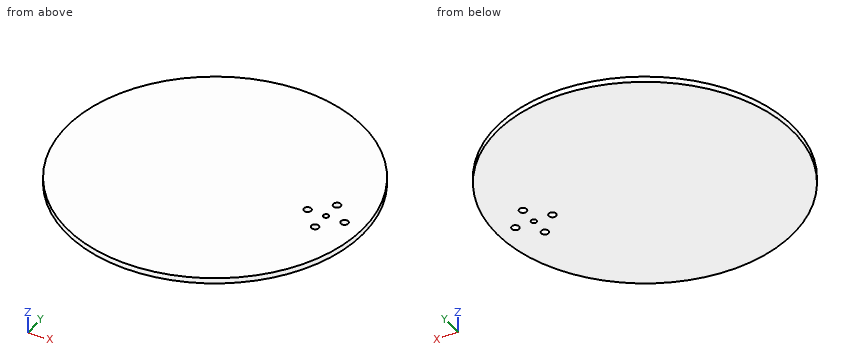
from build123d import *

# Parameters (mm, degrees)
SKETCH_1_R          = 80
EXTRUDE_1_DEPTH     = 3
SKETCH_2_R          = 2
SKETCH_2_R_2        = 1.5
CUT_EXTRUDE_4_DEPTH = 3


with BuildPart() as part:
    # 草图1 → 凸台-拉伸1 (new body)
    with BuildSketch(Plane.XY):
        Circle(SKETCH_1_R)
    extrude(amount=EXTRUDE_1_DEPTH)

    # 草图2 → 切除-拉伸4 (cut)
    with BuildSketch(Plane.XY.offset(3)):
        with Locations((70, 0)):
            Circle(SKETCH_2_R)
        with Locations((60, -10)):
            Circle(SKETCH_2_R)
        with Locations((60, 0)):
            Circle(SKETCH_2_R_2)
        with Locations((50, 0)):
            Circle(SKETCH_2_R)
        with Locations((60, 10)):
            Circle(SKETCH_2_R)
    extrude(amount=-CUT_EXTRUDE_4_DEPTH, mode=Mode.SUBTRACT)


solid = part.part
Geometry check sheet. Reference: the model listing, model coordinates, mm. Give positions to 0.01 mm unless a question says otherwise; leave off trailing zeros. Write each loop counter-clockwise with the first axis right and the second up, starting at its lowest first coordinate (ties: lowest second). Pieces come first, ordered by that corner, then holes. Notation, with made-up numbers: M -13.5,53 L 36.5,53 A31 ccw 36.5,90 Z; hole C 45.25,-26 d6. An arc over 180 degrees is marked long. One line per question, with ' | ' between items.
1. Cross-section at C-C (x = 70). Enter the section's corners in (y, z), plus the area to 3 significant figures.
Ans:
outline: M -38.73,0 L -2,0 L -2,3 L -38.73,3 Z; M 2,0 L 38.73,0 L 38.73,3 L 2,3 Z | area: 220 mm2
2. Cross-section at A-A (z = 1.55). Enter the section's corners in (x, y), plus the area to 3 significant figures.
Ans:
outline: C 0,0 d160; hole C 50,0 d4; hole C 60,-10 d4; hole C 60,10 d4; hole C 60,0 d3; hole C 70,0 d4 | area: 20,000 mm2
3. Scan lines: line 1 along Y through (x, z) = (60, 0.75); line 2 along Y through (x, z) = (70, 1.8); line 3 along X through (y, z) = (1, 1.55). Record each from-to range of solid material in increasing order. Write a range as from..to.
Ans:
line 1: -52.92..-12, -8..-1.5, 1.5..8, 12..52.92 | line 2: -38.73..-2, 2..38.73 | line 3: -79.99..48.27, 51.73..58.88, 61.12..68.27, 71.73..79.99
4. Cross-section at B-B (y = 10). Enter the section's corners in (x, z).
Ans:
outline: M -79.37,0 L 58,0 L 58,3 L -79.37,3 Z; M 62,0 L 79.37,0 L 79.37,3 L 62,3 Z
5. Cross-section at D-D (y = -63.5). Enter the section's corners in (x, z).
Ans:
outline: M -48.66,0 L 48.66,0 L 48.66,3 L -48.66,3 Z
6. Gauge pin test, flat ends, axial feed: pin 1 (2.5 mm diameter, centred on x = 60, y = 0, fed in from +Z); pin 2 (12 mm diameter, centred on x = 45.5, y = 15.5, fed in from -Z). Record the tip position at first contact, or that the pin passes through.
Ans:
pin 1: through | pin 2: z = 0
